Could you check a few things on this model? Use its own coordinates, in mm. Face numbers are marked on the shaded views. A direction names the side the tool comes from. Give positions to 0.01 mm unless a question says otherwise; leave off trailing zeros. Order: outer loops, then holes, each group sorted by start corner. A loop starts at its lowest first (then second) coordinate and runs counter-clockwise, first axis right, second up. Notation, with made-up numbers: (10.5, -14) - (68.5, -14) arc R28 ccw to (68.5, 14) - close; hole circle Ø6 at (7.5, 26). An arc over 180 degrees is marked (long way). One line per question, with ' | ' between items. Start each with the question number.
1. Which directions (+Z, -Z, +X, -X, +Y, -Y) give clear straight access to the entire face, cutting with the end or side of a thin tool? Please do the marked faces 1, 2, 3, 4 and 5.
2. Imagine slicing it at B-B (z = 104.5). Please give me the cut outline in (x, y).
3. I need wall thicknesses on probe 1 along X at (y, z) = (-0.5, 44); probe 2 along Z at (x, y) = (17, 5); probe 3 along Z at (x, y) = (4.5, 15.5). Which ranges of each line are inside material? Lowest first, please. Write a range as from..to.
4. For P1, Ø0.9, axis at x = 10, y = -12.5, coming from the +Z side; P2, Ø1.5, axis at x = 14, y = -14, coming from the +Z side; P3, Ø3.5, axis at x = -14.5, z = 10.5, coming from the +Y side; P4, Ø6, axis at y = -9, z = 103, coming from the +X side, each with a flat end and sliding along its axis, tell me the tip position at first contact or that it passes through.
5. Imagine slicing it at A-A (z = 48.5). Please give me the cut outline in (x, y), and give its area (3 significant figures).
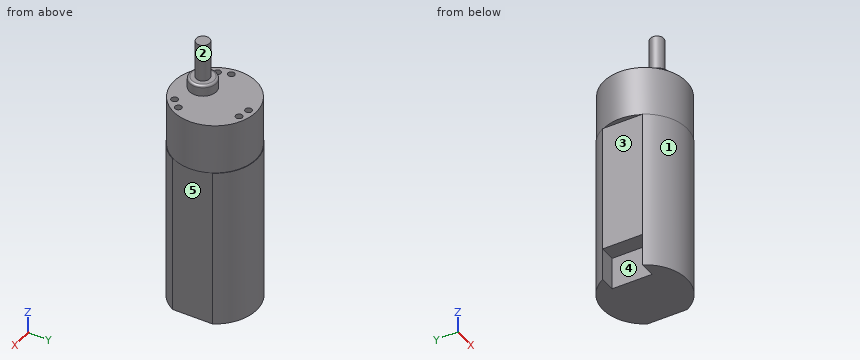
```python
from build123d import *

# Parameters (mm, degrees)
BOSS_EXTRUDE1_DEPTH = 72
SKETCH2_R           = 18.5
BOSS_EXTRUDE2_DEPTH = 22.5
SKETCH3_R           = 1.5
SKETCH3_R_2         = 6
CUT_EXTRUDE1_DEPTH  = 5
BOSS_EXTRUDE3_START = 10
SKETCH4_R           = 6
BOSS_EXTRUDE3_DEPTH = 10
FILLET1_R           = 1
SKETCH5_R           = 3
BOSS_EXTRUDE4_DEPTH = 17
SKETCH6_W           = 14.545544233
SKETCH6_H           = 17.81151313
CUT_EXTRUDE2_DEPTH  = 7


with BuildPart() as part:
    # Sketch1 → Boss-Extrude1 (new body)
    with BuildSketch(Plane.XY):
        with BuildLine():
            Line((-16.5, 8.905756565), (-16.5, -8.905756565))
            ThreePointArc((-16.5, -8.905756565), (0, -18.75), (16.5, -8.905756565))
            Line((16.5, -8.905756565), (16.5, 8.905756565))
            ThreePointArc((16.5, 8.905756565), (0, 18.75), (-16.5, 8.905756565))
        make_face()
    extrude(amount=BOSS_EXTRUDE1_DEPTH)

    # Sketch2 → Boss-Extrude2 (add)
    with BuildSketch(Plane.XY.offset(72)):
        with Locations(Location((0, 0, 0), (0, 0, 153.111952382))):
            Circle(SKETCH2_R)
    extrude(amount=BOSS_EXTRUDE2_DEPTH)

    # Sketch3 → Cut-Extrude1 (cut)
    with BuildSketch(Plane.XY.offset(94.5)):
        with Locations((-13.74680181, -7.160687119)):
            Circle(SKETCH3_R)
        with Locations((0.757881483, 15.430553719)):
            Circle(SKETCH3_R)
        with Locations((13.070128305, -8.426490905)):
            Circle(SKETCH3_R)
        with Locations((-15.366867454, -2.02716172)):
            Circle(SKETCH3_R)
        with Locations((5.92786018, 14.321678452)):
            Circle(SKETCH3_R)
        with Locations((9.439007274, -12.294516732)):
            Circle(SKETCH3_R)
        with Locations((-2.96393009, -7.160839226)):
            Circle(SKETCH3_R_2)
    extrude(amount=-CUT_EXTRUDE1_DEPTH, mode=Mode.SUBTRACT)

    # Sketch4 → Boss-Extrude3 (add)
    with BuildSketch(Plane.XY.offset(89.5).offset(BOSS_EXTRUDE3_START)):
        with Locations((-2.96393009, -7.160839226)):
            Circle(SKETCH4_R)
    extrude(amount=-BOSS_EXTRUDE3_DEPTH)

    # Fillet1
    fillet1_edges = [part.edges().sort_by_distance(p)[0] for p in [
        (-8.96393009, -7.160839226, 99.5),
    ]]
    fillet(fillet1_edges, radius=FILLET1_R)

    # Sketch5 → Boss-Extrude4 (add)
    with BuildSketch(Plane.XY.offset(99.5)):
        with Locations((-2.96393009, -7.160839226)):
            Circle(SKETCH5_R)
    extrude(amount=BOSS_EXTRUDE4_DEPTH)

    # Sketch6 → Cut-Extrude2 (cut)
    with BuildSketch(Plane.ZY.offset(16.5)):
        with Locations((7.272772117, 0)):
            Rectangle(SKETCH6_W, SKETCH6_H)
    extrude(amount=-CUT_EXTRUDE2_DEPTH, mode=Mode.SUBTRACT)


solid = part.part
```
Results found:
1) face 1: +Z, -Z, -Y | face 2: +Z | face 3: -Z, -X, +Y, -Y | face 4: -Z, -X | face 5: -Z, +X, +Y, -Y
2) outline: circle Ø6 at (-2.96, -7.16)
3) probe 1: x = -16.5..16.5 | probe 2: z = 72..94.5 | probe 3: z = 0..94.5
4) P1: stops at z = 89.5 | P2: passes through | P3: stops at y = 13.75 | P4: stops at x = 0.04
5) outline: (-16.5, -8.91) arc R18.75 ccw to (16.5, -8.91) - (16.5, 8.91) arc R18.75 ccw to (-16.5, 8.91) - close | area: 1,050 mm2
